Model file for the job. Use its own axes, mm. A direction names the side the tool comes from. Coordinates: 2 decimals unless noted, no trailing zeros. Loops run counter-clockwise (first coordinate to the right, second up) from the corner with the lowest first, then second, coordinate; pieces in that order, holes last.
from build123d import *

# Parameters (mm, degrees)
ESBO_O1_R                               = 3
RESSALTO_EXTRUS_O1_DEPTH                = 20
BROCA_DE_ROSQUEAR_PARA_TARRAXA_DE_M42_D = 3.3
CORTE_EXTRUS_O1_DEPTH                   = 50
CORTE_EXTRUS_O2_DEPTH                   = 50


with BuildPart() as part:
    # Esboço1 → Ressalto-extrusão1 (new body)
    with BuildSketch(Plane(origin=(0, 0, 0), x_dir=(0, 0, -1), z_dir=(1, 0, 0))):
        with BuildLine():
            Line((0, 0), (0, 5))
            Line((0, 5), (6.239506285, 5))
            ThreePointArc((6.239506285, 5), (8.431241444, 5.505970962), (10.179394863, 6.921481202))
            Line((10.179394863, 6.921481202), (40.043100593, 45.14105393))
            ThreePointArc((40.043100593, 45.14105393), (43.268998574, 47.25579782), (47.115650024, 46.969734684))
            Line((47.115650024, 46.969734684), (102.344683137, 23.522903311))
            ThreePointArc((102.344683137, 23.522903311), (105.522903311, 15.655316863), (97.655316863, 12.477096689))
            Line((97.655316863, 12.477096689), (50.195717148, 32.625507204))
            ThreePointArc((50.195717148, 32.625507204), (46.990174273, 32.86389315), (44.301925956, 31.101606576))
            Line((44.301925956, 31.101606576), (20, 0))
            Line((20, 0), (0, 0))
        make_face()
        with Locations((44.770966887, 41.446831372)):
            Circle(ESBO_O1_R, mode=Mode.SUBTRACT)
        with Locations((100, 18)):
            Circle(ESBO_O1_R, mode=Mode.SUBTRACT)
    extrude(amount=RESSALTO_EXTRUS_O1_DEPTH)

    # Broca de rosquear para tarraxa de M42 (through all)
    with Locations(Plane(origin=(0, 0, 0), x_dir=(-1, 0, 0), z_dir=(0, -1, 0))):
        with Locations((-10, 15), (-10, 5), (-5, 10), (-15, 10)):
            Hole(BROCA_DE_ROSQUEAR_PARA_TARRAXA_DE_M42_D / 2)

    # Esboço10 → Corte-extrusão1 (cut)
    with BuildSketch(Plane(origin=(0, 0, 0), x_dir=(1, 0, 0), z_dir=(0, 1, 0))):
        with BuildLine():
            Line((4.5, 36), (4.5, 73))
            ThreePointArc((4.5, 73), (5.671572875, 75.828427125), (8.5, 77))
            Line((8.5, 77), (11.5, 77))
            ThreePointArc((11.5, 77), (14.328427125, 75.828427125), (15.5, 73))
            Line((15.5, 73), (15.5, 36))
            ThreePointArc((15.5, 36), (14.328427125, 33.171572875), (11.5, 32))
            Line((11.5, 32), (8.5, 32))
            ThreePointArc((8.5, 32), (5.671572875, 33.171572875), (4.5, 36))
        make_face()
    extrude(amount=CORTE_EXTRUS_O1_DEPTH, mode=Mode.SUBTRACT)

    # Esboço11 → Corte-extrusão2 (cut)
    with BuildSketch(Plane(origin=(0, 0, 0), x_dir=(1, 0, 0), z_dir=(0, 1, 0))):
        with BuildLine():
            Line((5, 106), (5, 88.5))
            ThreePointArc((5, 88.5), (5.732233047, 86.732233047), (7.5, 86))
            Line((7.5, 86), (12.5, 86))
            ThreePointArc((12.5, 86), (14.267766953, 86.732233047), (15, 88.5))
            Line((15, 88.5), (15, 106))
            Line((15, 106), (5, 106))
        make_face()
    extrude(amount=CORTE_EXTRUS_O2_DEPTH, mode=Mode.SUBTRACT)


solid = part.part
Q1. Slice it at B-B (z = -5). List the corners of the cut face in (x, y).
Answers:
outline: (0, 0) - (8.35, 0) - (8.35, 5) - (0, 5) - close; (11.65, 0) - (20, 0) - (20, 5) - (11.65, 5) - close
Q2. Mould opens along Y. For faces 6 (the cylindrical face through (17.5, 16.2, -97.6)), 7 (the cylindrical face through (2.465, 15.777, -105.573)), 8 (the flat face through (10, 0, -10)) say: +Y half, -Y half, draft (parallel to the pull), parting line (faces both ways), or undercut.
Answers:
face 6: undercut
face 7: parting line
face 8: -Y half
Q3. Slice it at C-C (y = 43.5). List the corners of the cut face in (x, z).
Answers:
outline: (0, -55.29) - (4.5, -55.29) - (4.5, -46.96) - (0, -46.96) - close; (0, -42.58) - (4.5, -42.58) - (4.5, -38.76) - (0, -38.76) - close; (15.5, -55.29) - (20, -55.29) - (20, -46.96) - (15.5, -46.96) - close; (15.5, -42.58) - (20, -42.58) - (20, -38.76) - (15.5, -38.76) - close
Q4. Drill centre lines: line 1 (X direction, y = 3, z = -10); line 2 (X direction, y = 1.9, z = -5); line 3 (Z direction, x = 18.95, y = 18). Where is each one in solid material? Low to high.
Answers:
line 1: x = 0 to 3.35, 6.65 to 13.35, 16.65 to 20
line 2: x = 0 to 8.35, 11.65 to 20
line 3: z = -106 to -103, -97 to -84.65, -34.06 to -18.84
Q5. Flat gauge pins, fed straight in: P1, Ø3, axis at x = 17, z = -76.5, coming from the +Y side; P2, Ø4.5, axis at x = 15, z = -10, coming from the +Y side; P3, Ø3, axis at x = 11.5, z = -4.5, coming from the +Y side. Where does each tip first touch, or does it go through?
Answers:
P1: stops at y = 35.13
P2: stops at y = 9.57
P3: stops at y = 5
Q6. Slice it at A-A (z = -100). List the corners of the cut face in (x, y).
Answers:
outline: (0, 12) - (5, 12) - (5, 15) - (0, 15) - close; (0, 21) - (5, 21) - (5, 24.52) - (0, 24.52) - close; (15, 12) - (20, 12) - (20, 15) - (15, 15) - close; (15, 21) - (20, 21) - (20, 24.52) - (15, 24.52) - close
Q7. Slice it at D-D (z = -66). List the corners of the cut face in (x, y).
Answers:
outline: (0, 25.92) - (4.5, 25.92) - (4.5, 38.95) - (0, 38.95) - close; (15.5, 25.92) - (20, 25.92) - (20, 38.95) - (15.5, 38.95) - close
Q8. Which spindle directions (+Z, -Z, +X, -X, +Y, -Y) get a long thin tool onto all of the face, cutting with end or side? Do faces 1 (the flat face through (10, 5, -3)), 2 (the cylindrical face through (5.713, 23.314, -86.752)), 3 (the cylindrical face through (2.5, 16.2, -97.6)), 4 (the cylindrical face through (14.297, 28.51, -75.859)), 5 (the flat face through (9.86, 12.31, -29.62)). Say none if no direction does.
Answers:
face 1: +Z, +X, -X, +Y
face 2: -Z, +Y, -Y
face 3: +X, -X
face 4: +Y, -Y
face 5: +X, -X, -Y
